For this review, take the finished solid that the model builds, in its own axes (mm). Coordinates: 2 decimals unless noted, no trailing zeros. Loops run counter-clockwise (first coordinate to the right, second up) from the corner with the lowest first, then second, coordinate; pieces in that order, holes last. Notation, with made-up numbers: (-16, 72) - (-7, 72) arc R21 cw to (-7, 106) - close; hole circle Ø1 at (-28, 65). An arc over 180 degrees is marked (long way). Use one line per item in the form item = value. Start each with the question number.
1. For pin 1 Ø3 at (x, z) = (0, 3.5) entering from -Y; pin 2 Ø2 at (x, y) = (-3, 32) entering from +Z, all flat-tipped, find the tip position at first contact; note any pin that passes through.
2. Add section A-A on z = 0. Give the boundary of the cut face in (x, y) (3 decimals), and give its area (3 significant figures).
3. Add section C-C on x = 0. Give the boundary of the cut face in (y, z) (3 decimals), and give its area (3 significant figures).
4. To check wall thickness, follow probe 1 along X at (y, z) = (21.5, 0); probe 2 along Z at (x, y) = (-2.25, 5); probe 3 along Z at (x, y) = (-2, 21). State the ranges of each line that lie inside material, in increasing order.
5. Add section D-D on z = -6. Give the boundary of the cut face in (x, y) (3 decimals).
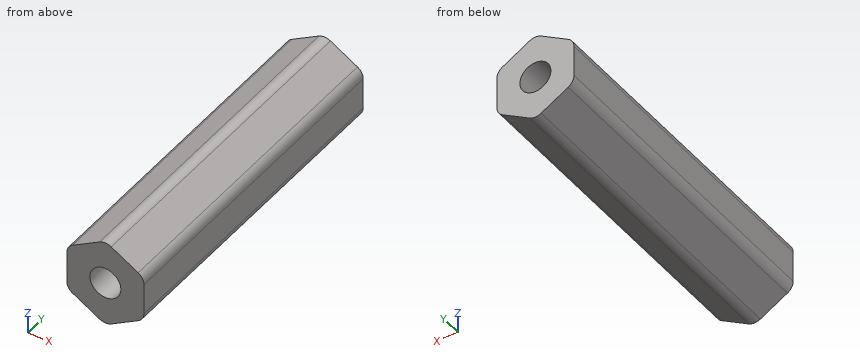
```python
from build123d import *

# Parameters (mm, degrees)
SKETCH1_R           = 2.5527
BOSS_EXTRUDE1_DEPTH = 53.975
FILLET1_R           = 1.905


with BuildPart() as part:
    # Sketch1 → Boss-Extrude1 (new body)
    with BuildSketch(Plane(origin=(0, 0, 0), x_dir=(1, 0, 0), z_dir=(0, 1, 0))):
        Polygon((0, 7.332348419), (-6.35, 3.666174209), (-6.35, -3.666174209), (0, -7.332348419), (6.35, -3.666174209), (6.35, 3.666174209), align=None)
        with Locations(Location((0, 0, 0), (0, 0, 270))):
            Circle(SKETCH1_R, mode=Mode.SUBTRACT)
    extrude(amount=BOSS_EXTRUDE1_DEPTH)

    # Fillet1
    fillet1_edges = [part.edges().sort_by_distance(p)[0] for p in [
        (6.35, 26.9875, -3.666174209),
        (6.35, 26.9875, 3.666174209),
        (0, 26.9875, 7.332348419),
        (-6.35, 26.9875, 3.666174209),
        (-6.35, 26.9875, -3.666174209),
        (0, 26.9875, -7.332348419),
    ]]
    fillet(fillet1_edges, radius=FILLET1_R)


solid = part.part
```
Conclusion:
q1.pin_1 = 0
q1.pin_2 = 6.18
q2.outline = (-6.35, 0) - (-2.553, 0) - (-2.553, 53.975) - (-6.35, 53.975) - close; (2.553, 0) - (6.35, 0) - (6.35, 53.975) - (2.553, 53.975) - close
q2.area = 410 mm^2
q3.outline = (0, -7.038) - (53.975, -7.038) - (53.975, -2.553) - (0, -2.553) - close; (0, 2.553) - (53.975, 2.553) - (53.975, 7.038) - (0, 7.038) - close
q3.area = 484 mm^2
q4.probe_1 = -6.35 to -2.55, 2.55 to 6.35
q4.probe_2 = -6.03 to -1.21, 1.21 to 6.03
q4.probe_3 = -6.18 to -1.59, 1.59 to 6.18
q5.outline = (-2.308, 0) - (2.308, 0) - (2.308, 53.975) - (-2.308, 53.975) - close
